Design review of the part built by this model. Coordinates are the model's own, in mm. A direction names the side the tool comes from. Coordinates: 2 decimals unless noted, no trailing zeros. Write each loop counter-clockwise with the first axis right and the second up, starting at its lowest first coordinate (ties: lowest second). Pieces come first, ordered by that corner, then holes.
Q1. Take a section at A-A, the plane x = 5.2. Write out the cut boundary in (y, z).
Q2. For L1, parallel to Z at x = 1.25, y = -1.6; L2, parallel to X at y = -1.4, z = 2; L3, parallel to X at y = -1.4, z = 9, list the stretches that pass through material, from the lowest coordinate up.
Q3. Take a section at B-B, the plane z = 6.5. Write out the cut boundary in (x, y), plus the area to 3 significant figures.
Q4. The part is to be moulded in two halves that separate along Z. For faces 1 (the flat face through (5, -3, -2)), 2 (the flat face through (-2, -3, 4)), 3 (the flat face through (0, -3, 2)), say which applies: released by +Z, released by -Z, zero draft, split by the parting line, or undercut.
Q5. For pin 1 Ø1.8 at (x, y) = (5, -3) entering from +Z (3 decimals); pin 2 Ø2 at (x, y) = (3, -3) entering from +Z, all flat-tipped, find the tip position at first contact; note any pin that passes through.
Q6. For faces 4 (the flat face through (2.7, -3, 9)), 5 (the flat face through (10.4, -3, 2)), 6 (the flat face through (5, -6, 5)), list the 3-axis set-ups (+Z, -Z, +X, -X, +Y, -Y) from which the entire face can be reached by the end or side of a thin tool; tool diameter is ignored.
Q7. Take a section at C-C, the plane y = -5.05. Write out the cut boundary in (x, z), plus the area to 3 significant figures.
from build123d import *

# Parameters (mm, degrees)
F0_W     = 10.4
F0_H     = 4.2
F1_DEPTH = 6


with BuildPart() as f1:
    # F0 (on Front) → F1 (new body)
    with BuildSketch(Plane.XZ):
        with BuildLine():
            Line((-2, 6), (-2, -2))
            Line((-2, -2), (12.4, -2))
            Line((12.4, -2), (12.4, 6))
            Line((12.4, 6), (12.4, 8.5))
            Line((12.4, 8.5), (12.4, 9.47713))
            Line((12.4, 9.47713), (7.7, 9.47713))
            Line((7.7, 9.47713), (7.7, 8.5))
            ThreePointArc((7.7, 8.5), (5.2, 6), (2.7, 8.5))
            Line((2.7, 8.5), (2.7, 9.47713))
            Line((2.7, 9.47713), (-2, 9.47713))
            Line((-2, 9.47713), (-2, 8.5))
            Line((-2, 8.5), (-2, 6))
        make_face()
        with Locations((5.2, 2.1)):
            Rectangle(F0_W, F0_H, mode=Mode.SUBTRACT)
    extrude(amount=F1_DEPTH)


solid = f1.part
Responses:
1. outline: (-6, -2) - (0, -2) - (0, 0) - (-6, 0) - close; (-6, 4.2) - (0, 4.2) - (0, 6) - (-6, 6) - close
2. L1: z = -2 to 0, 4.2 to 9.48
2. L2: x = -2 to 0, 10.4 to 12.4
2. L3: x = -2 to 2.7, 7.7 to 12.4
3. outline: (-2, -6) - (3.7, -6) - (3.7, 0) - (-2, 0) - close; (6.7, -6) - (12.4, -6) - (12.4, 0) - (6.7, 0) - close
3. area: 68.4 mm2
4. face 1: released by -Z
4. face 2: zero draft
4. face 3: undercut
5. pin 1: stops at z = 6.255
5. pin 2: stops at z = 9.48
6. face 4: +Z, +Y, -Y
6. face 5: +Y, -Y
6. face 6: +Z, -Z, +X, -X, -Y
7. outline: (-2, -2) - (12.4, -2) - (12.4, 9.48) - (7.7, 9.48) - (7.7, 8.5) arc R2.5 cw to (2.7, 8.5) - (2.7, 9.48) - (-2, 9.48) - close; hole (0, 0) - (10.4, 0) - (10.4, 4.2) - (0, 4.2) - close
7. area: 107 mm2
